Could you check a few things on this model? Use its own coordinates, in mm. Face numbers are marked on the shaded views. Coordinates: 2 decimals unless noted, no trailing zeros. Write each loop counter-clockwise with the first axis right and the second up, starting at its lowest first coordinate (ties: lowest second). Pieces come first, ordered by that corner, then holes.
Item 1: I want a section at A-A on z = 8.4. Please give me the cut outline in (x, y).
Item 2: Thinking about a two-plate mould opening in X: for the marked faces 1, 2, 3 and 4, which applies, +X half, -X half, draft (parallel to the pull), parting line (faces both ways), or undercut?
Item 3: If I drill on probe 1 along X at (y, z) = (1, 8.4); probe 2 along X at (y, z) = (-1.5, 7.25); probe 3 along Z at (x, y) = (-0.25, -0.5), over which ranges is the centre line in solid material (lowest first)?
Item 4: I want a section at B-B on y = 3.25. Please give me the cut outline in (x, z).
Item 5: I want a section at C-C on x = 0. Please give me the cut outline in (y, z), then the cut area to 3 significant figures.
from build123d import *

# Parameters (mm, degrees)
BOSS_EXTRUDE1_DEPTH      = 10
BOSS_EXTRUDE1_DEPTH_BACK = 5
SKETCH1_W                = 7.5
SKETCH1_H                = 10
SKETCH2_R                = 2.2
CUT_EXTRUDE1_DEPTH       = 14.462912018
FILLET1_R                = 0.6


with BuildPart() as part:
    # Sketch1 → Boss-Extrude1 (new, two sides: drawn at the far end of the back side and taken through both)
    with BuildSketch(Plane(origin=(0, 0, 0), x_dir=(0, 1, 0), z_dir=(0, 0, 1)).offset(-BOSS_EXTRUDE1_DEPTH_BACK)):
        Rectangle(SKETCH1_W, SKETCH1_H)
    extrude(amount=BOSS_EXTRUDE1_DEPTH + BOSS_EXTRUDE1_DEPTH_BACK)

    # Sketch2 → Cut-Extrude1 (cut, through all)
    with BuildSketch(Plane(origin=(0, 3.75, 0), x_dir=(-1, 0, 0), z_dir=(0, 1, 0))):
        with Locations((0, 8.4)):
            Circle(SKETCH2_R)
    extrude(amount=-CUT_EXTRUDE1_DEPTH, mode=Mode.SUBTRACT)

    # Fillet1
    fillet1_edges = [part.edges().sort_by_distance(p)[0] for p in [
        (-5, 0, 10),
        (5, 0, 10),
        (-1.509966887, 0, 10),
        (1.509966887, 0, 10),
    ]]
    fillet(fillet1_edges, radius=FILLET1_R)


solid = part.part
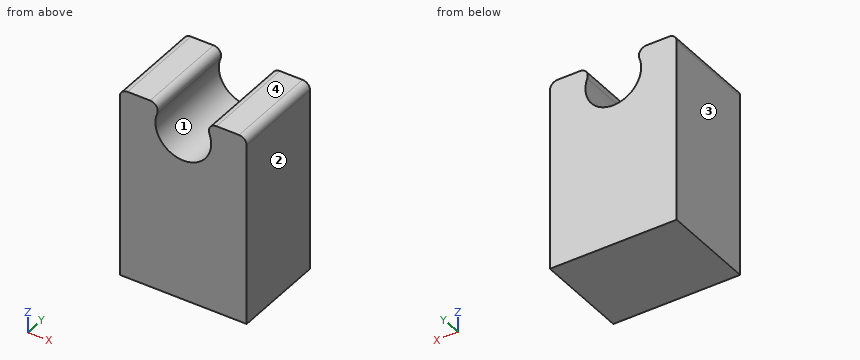
Response values:
1. outline: (-5, -3.75) - (-2.2, -3.75) - (-2.2, 3.75) - (-5, 3.75) - close; (2.2, -3.75) - (5, -3.75) - (5, 3.75) - (2.2, 3.75) - close
2. face 1: undercut
2. face 2: +X half
2. face 3: -X half
2. face 4: draft
3. probe 1: x = -5 to -2.2, 2.2 to 5
3. probe 2: x = -5 to -1.88, 1.88 to 5
3. probe 3: z = -5 to 6.21
4. outline: (-5, -5) - (5, -5) - (5, 9.4) arc R0.6 ccw to (4.4, 10) - (2.62, 10) arc R0.6 ccw to (2.05, 9.19) arc R2.2 cw (long way) to (-2.05, 9.19) arc R0.6 ccw to (-2.62, 10) - (-4.4, 10) arc R0.6 ccw to (-5, 9.4) - close
5. outline: (-3.75, -5) - (3.75, -5) - (3.75, 6.2) - (-3.75, 6.2) - close
5. area: 84.0 mm2
